Drawing for the job (mm, zero at the part's lowest x, y, z). A direction names the side the tool comes from. Give positions to 0.01 mm unless a question says otherwise; leave off trailing zeros. Order: outer loops, then holes, each group sorted by start corner. A loop starts at its lowest first (then second) coordinate and runs counter-clockwise, first axis right, second up. Notation, with made-up numbers: M -38,12.5 L 9,12.5 A13 cw 9,16.5 Z; hole C 59.5,-24 d6. An arc over 180 degrees is marked long. Answer as a JSON object with one key per item and string values.
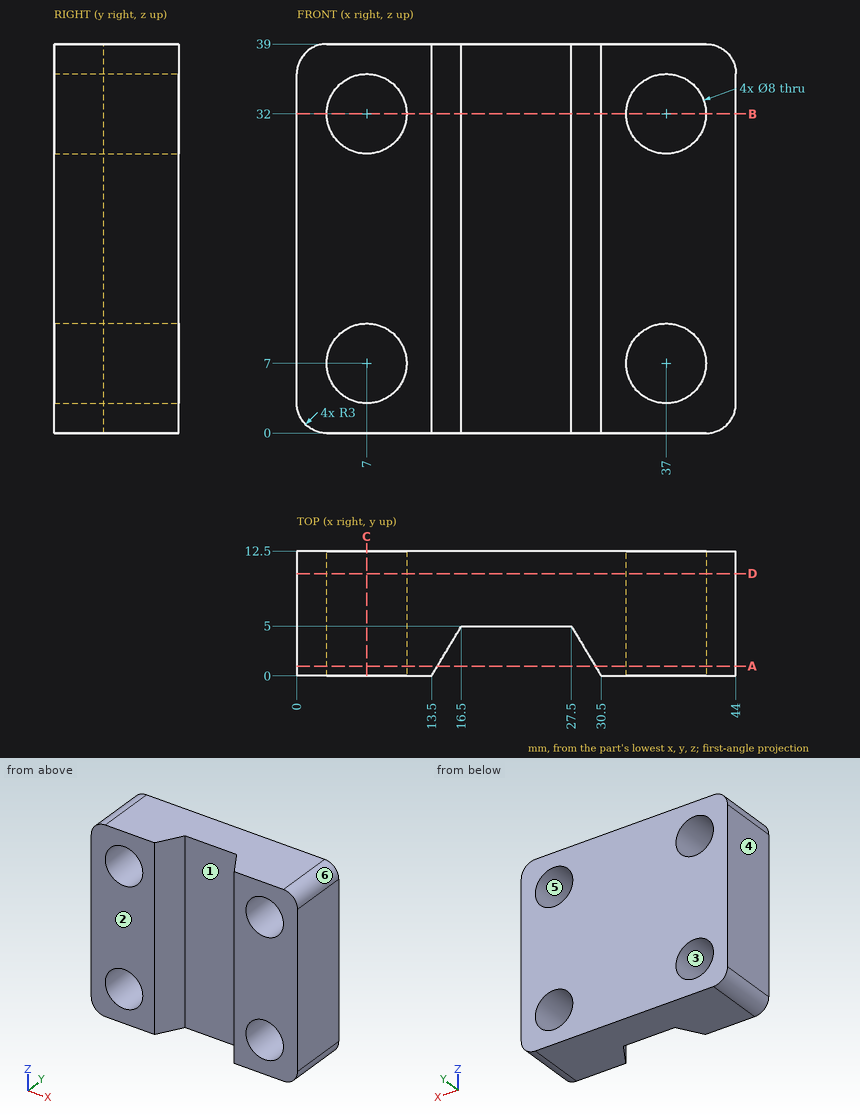
1. Two-plate mould, pull along Z, no slides. Class the marked faces 3, 4, 5 and 6: +Z half, -Z half, draft (parallel to the pull), parting line (faces both ways), or undercut.
Worked answers:
{"face 3": "undercut", "face 4": "draft", "face 5": "undercut", "face 6": "+Z half"}
2. Probe line 1 along Z through (x, y) = (37, 5.75); line 2 along X through (y, z) = (8.25, 7); line 3 along Z through (x, y) = (34, 9.5). List the from-to ranges inside material, lowest first.
Worked answers:
{"line 1": "z = 0 to 3, 11 to 28, 36 to 39", "line 2": "x = 0 to 3, 11 to 33, 41 to 44", "line 3": "z = 0 to 4.35, 9.65 to 29.35, 34.65 to 39"}
3. Cut at B-B on z = 32. Give the cut face in (x, y).
Worked answers:
{"outline": "M 0,0 L 3,0 L 3,12.5 L 0,12.5 Z; M 11,0 L 13.5,0 L 16.5,5 L 27.5,5 L 30.5,0 L 33,0 L 33,12.5 L 11,12.5 Z; M 41,0 L 44,0 L 44,12.5 L 41,12.5 Z"}
4. Cut at C-C on x = 7. Give the cut face in (y, z), plus the area to 4 significant figures.
Worked answers:
{"outline": "M 0,0 L 12.5,0 L 12.5,3 L 0,3 Z; M 0,11 L 12.5,11 L 12.5,28 L 0,28 Z; M 0,36 L 12.5,36 L 12.5,39 L 0,39 Z", "area": "287.5 mm^2"}
5. Which spindle directions (+Z, -Z, +X, -X, +Y, -Y) get a long thin tool onto all of the face, cutting with end or side? Do the marked faces 1 and 2. Say none if no direction does.
Worked answers:
{"face 1": "+Z, -Z, -Y", "face 2": "+Z, -Z, +X, -X, -Y"}
6. Pin check, flat tips, straight feed: P1, Ø12, axis at x = 22.5, z = 22.5, coming from the -Y side; P2, Ø12, axis at x = 23.5, z = 6.5, coming from the -Y side. Stop position of each tip, or through.
Worked answers:
{"P1": "stops at y = 3.33", "P2": "stops at y = 1.67"}
7. Cut at D-D on y = 10.25. Give the cut face in (x, z).
Worked answers:
{"outline": "M 0,3 A3 ccw 3,0 L 41,0 A3 ccw 44,3 L 44,36 A3 ccw 41,39 L 3,39 A3 ccw 0,36 Z; hole C 7,7 d8; hole C 7,32 d8; hole C 37,7 d8; hole C 37,32 d8"}
8. Cut at A-A on y = 1. Give the cut face in (x, z), plus the area to 3 significant figures.
Worked answers:
{"outline": "M 0,3 A3 ccw 3,0 L 14.1,0 L 14.1,39 L 3,39 A3 ccw 0,36 Z; M 29.9,0 L 41,0 A3 ccw 44,3 L 44,36 A3 ccw 41,39 L 29.9,39 Z; hole C 7,7 d8; hole C 7,32 d8; hole C 37,7 d8; hole C 37,32 d8", "area": "891 mm^2"}
